Work out the finished part from the listing and answer in its coordinate system (mm). Round coordinates to 2 decimals unless told otherwise and drop trailing zeros. Order: outer loops, then holes, each group sorted by start corner. A loop starts at its lowest first (then second) coordinate and runs counter-clockwise, first axis right, second up. Notation, with made-up numbers: (7, -2) - (13, -2) arc R27 ccw to (13, 36) - close; hole circle Ø3 at (43, 30). An arc over 180 degrees is marked (long way). Put each result on its own line as item: value.
```python
from build123d import *

# Parameters (mm, degrees)
F0_R     = 15
F1_DEPTH = 25


with BuildPart() as f1:
    # F0 (on Top) → F1 (new body)
    with BuildSketch(Plane.XY):
        Polygon((-20.309781, -21.567568), (20.309781, -21.567568), (27.385138, -14.834567), (27.385138, 14.834567), (20.309781, 21.567568), (-20.309781, 21.567568), (-27.385138, 14.834567), (-27.385138, -14.834567), align=None)
        Circle(F0_R, mode=Mode.SUBTRACT)
    extrude(amount=F1_DEPTH)


solid = f1.part
```
1) A cutting plane is placed at C-C on z = 10.75. Write down the section's boundary in (x, y), then the cut area to 3 significant figures.
Findings below:
outline: (-27.39, -14.83) - (-20.31, -21.57) - (20.31, -21.57) - (27.39, -14.83) - (27.39, 14.83) - (20.31, 21.57) - (-20.31, 21.57) - (-27.39, 14.83) - close; hole circle Ø30 at (0, 0)
area: 1,560 mm2
2) A cutting plane is placed at B-B on x = 0. Write down the section's boundary in (y, z), then the cut area to 3 significant figures.
Findings below:
outline: (-21.57, 0) - (-15, 0) - (-15, 25) - (-21.57, 25) - close; (15, 0) - (21.57, 0) - (21.57, 25) - (15, 25) - close
area: 328 mm2
3) For a pull along Y with two mould halves and no side action, classify faces 1 (the flat face through (-27.385, 0, 12)), 2 (the cylindrical face through (-14.985, 0.66, 12.325)), 3 (the flat face through (23.798, -18.248, 12.325)) as pulls with the +Y half, pulls with the -Y half, needs draft (parallel to the pull), parting line crosses it, or undercut.
Findings below:
face 1: needs draft
face 2: undercut
face 3: pulls with the -Y half
4) A cutting plane is placed at A-A on y = 0. Write down the section's boundary in (x, z).
Findings below:
outline: (-27.39, 0) - (-15, 0) - (-15, 25) - (-27.39, 25) - close; (15, 0) - (27.39, 0) - (27.39, 25) - (15, 25) - close
5) Straight lines are drawn through the part: L1, parallel to Y at x = 0.5, z = 6.25; L2, parallel to X at y = -9.5, z = 7; L3, parallel to X at y = 11, z = 5. For each, find the intervals that lie inside material, in ascending order. Write a range as from..to.
Findings below:
L1: y = -21.57..-14.99, 14.99..21.57
L2: x = -27.39..-11.61, 11.61..27.39
L3: x = -27.39..-10.2, 10.2..27.39
